Autodesk Inventor part; units mm, degrees
ref_plane "Work Plane1" through (-56.3599, 0, 22) normal (0, 0, -1) x (-1, 0, 0)
ref_plane "YZ Plane" through (0, 0, 0) normal (1, 0, 0) x (0, 1, 0)
ref_plane "XZ Plane" through (0, 0, 0) normal (0, 1, 0) x (-1, 0, 0)
ref_plane "Work Plane1" through (-56.3599, 0, 22) normal (0, 0, -1) x (-1, 0, 0)
sketch "Sketch1" plane through (-56.3599, 0, 22) normal (0, 0, -1) x (-1, 0, 0)
  line L0 (-4.0299, -0.3538) -> (-2.2322, 1.4439) construction
  arc A0 (-1.4439, 2.2322) -> (-2.2322, 1.4439) centre (-0.9299, 0.9299) ccw construction
  line L1 (-1.4439, 2.2322) -> (0.3538, 4.0299) construction
  line L2 (-37.8299, 42.8299) -> (-37.8299, 37.8299) construction
  line L3 (-37.8299, 37.8299) -> (-42.9208, 37.8299) construction
  line L4 (-37.8299, 42.2137) -> (-37.8299, 45.8299) construction
  line L5 (-37.8299, 45.8299) -> (-4.0299, 45.8299) construction
  line L6 (-4.0299, 45.8299) -> (-4.0299, 42.2137) construction
  line L7 (-4.0299, 4.0299) -> (0.3538, 4.0299)
  circle A1 centre (-20.9299, 20.9299) radius 17.5
  line L8 (-20.9299, 58.9723) -> (17.1124, 20.9299) construction
  line L9 (17.1124, 20.9299) -> (-20.9299, -17.1124) construction
  line L10 (-20.9299, -17.1124) -> (-58.9723, 20.9299) construction
  line L11 (-58.9723, 20.9299) -> (-20.9299, 58.9723) construction
  line L12 (-20.9299, 58.9723) -> (-20.9299, -17.1124) construction
  line L13 (17.1124, 20.9299) -> (-58.9723, 20.9299) construction
  line L14 (-20.9299, 58.9723) -> (32.8701, 58.9723) construction
  line L15 (-43.4299, 43.4299) -> (1.5701, 43.4299) construction
  line L16 (1.5701, 43.4299) -> (1.5701, -1.5701) construction
  line L17 (1.5701, -1.5701) -> (-43.4299, -1.5701) construction
  line L18 (-43.4299, -1.5701) -> (-43.4299, 43.4299) construction
  line L19 (-43.4299, 43.4299) -> (1.5701, -1.5701) construction
  line L20 (1.5701, 43.4299) -> (-43.4299, -1.5701) construction
  line L21 (-43.4299, 5.3876) -> (-43.4299, 36.4723)
  line L22 (-43.4299, 36.4723) -> (-36.4723, 43.4299)
  line L23 (-36.4723, 43.4299) -> (-5.3876, 43.4299)
  line L24 (-5.3876, 43.4299) -> (1.5701, 36.4723)
  line L25 (1.5701, 36.4723) -> (1.5701, 5.3876)
  line L26 (1.5701, 5.3876) -> (-5.3876, -1.5701)
  line L27 (-5.3876, -1.5701) -> (-36.4723, -1.5701)
  line L28 (-36.4723, -1.5701) -> (-43.4299, 5.3876)
  line L29 (-4.0299, 42.2137) -> (-37.8299, 42.2137)
  line L30 (-4.0299, -0.3538) -> (-4.0299, 4.0299)
  circle A2 centre (-20.9299, 20.9299) radius 1.5
  line L31 (-10.9299, 10.9299) -> (-30.9299, 10.9299) construction
  line L32 (-30.9299, 10.9299) -> (-30.9299, 30.9299) construction
  line L33 (-30.9299, 30.9299) -> (-10.9299, 30.9299) construction
  line L34 (-10.9299, 30.9299) -> (-10.9299, 10.9299) construction
  line L35 (-10.9299, 10.9299) -> (-30.9299, 30.9299) construction
  line L36 (-30.9299, 10.9299) -> (-10.9299, 30.9299) construction
  circle A3 centre (-30.9299, 30.9299) radius 1.4
  circle A4 centre (-30.9299, 10.9299) radius 1.4
  circle A5 centre (-10.9299, 10.9299) radius 1.4
  line L37 (-45.8299, 37.8299) -> (-42.0723, 37.8299) construction
  line L38 (-42.1723, 37.7299) -> (-45.8299, 37.7299)
  line L39 (-45.8299, 37.7299) -> (-45.8299, 4.1299)
  line L40 (-45.8299, 4.1299) -> (-42.1723, 4.1299)
  line L41 (-42.1723, 4.1299) -> (-42.1723, 37.7299)
  line L42 (-45.8299, 4.0299) -> (-42.0723, 4.0299) construction
  line L43 (-45.8299, 37.8299) -> (-42.0723, 37.8299)
  line L44 (-37.7299, 45.8299) -> (-4.1299, 45.8299)
  line L45 (-4.1299, 45.8299) -> (-4.1299, 42.1723)
  line L46 (-4.1299, 42.1723) -> (-37.7299, 42.1723)
  line L47 (-37.7299, 42.1723) -> (-37.7299, 45.8299)
  line L48 (0.4701, 37.8299) -> (0.4701, 4.0299) construction
  line L49 (0.4701, 4.0299) -> (3.9701, 4.0299) construction
  line L50 (3.9701, 37.8299) -> (3.9701, 4.0299) construction
  line L51 (0.4701, 37.8299) -> (3.9701, 37.8299) construction
  line L52 (-45.8299, -3.9701) -> (-4.0299, -3.9701) construction
  line L53 (0.3124, 37.7299) -> (3.9701, 37.7299)
  line L54 (3.9701, 37.7299) -> (3.9701, 4.1299)
  line L55 (3.9701, 4.1299) -> (0.3124, 4.1299)
  line L56 (0.3124, 4.1299) -> (0.3124, 37.7299)
  line L57 (-4.1713, -0.3538) -> (-37.7299, -0.3538)
  line L58 (-37.7299, -0.3538) -> (-37.7299, -3.9701)
  line L59 (-37.7299, -3.9701) -> (-4.1713, -3.9701)
  line L60 (-4.1713, -3.9701) -> (-4.1713, -0.3538)
  point P0 (-37.8299, 4.0299)
  dimension "d18" = 53.8
  dimension "d19" = 45
  dimension "d20" = 53.8
  dimension "d21" = 45
  dimension "d22" = 45
  dimension "d30" = 20
  dimension "d31" = 20
  dimension "d32" = 2.8
  dimension "d33" = 2.8
  dimension "d34" = 2.8
  dimension "d35" = 3
  dimension "d36" = 0.1
  dimension "d37" = 0.1
  dimension "d38" = 0.1
  dimension "d39" = 0.1
extrude "Extrusion1" add sketch "Sketch1" along normal blind 8 contours L30 L26 L57 L28 L41 L22 L46 L24 L56 L7 | L7 L26 L30 | L56 L24 L25 L26 | L26 L25 L24 L53 L54 L55 | L60 L59 L58 L57 L28 L27 L26 | L26 L27 L28 L57 | L46 L22 L29 L24 | L24 L29 L45 | L40 L39 L38 L22 L21 L28 | L28 L21 L22 L41 | L29 L22 L23 L24 | L24 L23 L22 L29 L47 L44 L45 | L47 L29 L22 | A1 | A2 | A3 | A4 | A5
sketch "Skizze4" plane through (-56.3599, 0, 14) normal (0, 0, -1) x (-1, 0, 0)
  line L0 (-37.7299, 42.1723) -> (-42.1723, 37.7299)
  line L1 (-42.1723, 37.7299) -> (-45.8299, 37.7299)
  line L2 (-45.8299, 37.7299) -> (-45.8299, 4.1299) construction
  line L3 (-45.8299, 4.1299) -> (-42.1723, 4.1299)
  line L4 (-42.1723, 4.1299) -> (-37.6885, -0.3538)
  line L5 (-37.6885, -0.3538) -> (-37.7299, -0.3538)
  line L6 (-37.7299, -0.3538) -> (-37.7299, -3.9701)
  line L7 (-37.7299, -3.9701) -> (-4.1713, -3.9701) construction
  line L8 (-4.1713, -3.9701) -> (-4.1713, -0.3538)
  line L9 (-4.1713, -0.3538) -> (0.3124, 4.1299)
  line L10 (0.3124, 4.1299) -> (3.9701, 4.1299)
  line L11 (3.9701, 4.1299) -> (3.9701, 37.7299) construction
  line L12 (3.9701, 37.7299) -> (0.3124, 37.7299)
  line L13 (0.3124, 37.7299) -> (-4.1299, 42.1723)
  line L14 (-4.1299, 42.1723) -> (-4.1299, 45.8299)
  line L15 (-4.1299, 45.8299) -> (-37.7299, 45.8299) construction
  line L16 (-37.7299, 45.8299) -> (-37.7299, 42.1723)
  line L17 (-37.9299, 46.0299) -> (-3.9299, 46.0299) construction
  line L18 (-3.9299, 46.0299) -> (-3.9299, 42.2551)
  line L19 (-3.9299, 42.2551) -> (0.3953, 37.9299)
  line L20 (0.3953, 37.9299) -> (4.1701, 37.9299)
  line L21 (4.1701, 37.9299) -> (4.1701, 3.9299) construction
  line L22 (4.1701, 3.9299) -> (0.3953, 3.9299)
  line L23 (0.3953, 3.9299) -> (-3.9713, -0.4367)
  line L24 (-3.9713, -0.4367) -> (-3.9713, -4.1701)
  line L25 (-3.9713, -4.1701) -> (-37.9299, -4.1701) construction
  line L26 (-37.9299, -4.1701) -> (-37.9299, -0.3953)
  line L27 (-37.9299, -0.3953) -> (-42.2551, 3.9299)
  line L28 (-42.2551, 3.9299) -> (-46.0299, 3.9299)
  line L29 (-46.0299, 3.9299) -> (-46.0299, 37.9299) construction
  line L30 (-46.0299, 37.9299) -> (-42.2551, 37.9299)
  line L31 (-42.2551, 37.9299) -> (-37.9299, 42.2551)
  line L32 (-37.9299, 42.2551) -> (-37.9299, 46.0299)
  line L33 (-45.8299, 37.7299) -> (-45.8299, 37.9299)
  line L34 (-4.1299, 45.8299) -> (-37.7299, 45.8299)
  line L35 (-37.7299, 45.8299) -> (-37.9299, 45.8299)
  line L36 (-4.1299, 45.8299) -> (-3.9299, 45.8299)
  line L37 (3.9701, 37.7299) -> (3.9701, 37.9299)
  line L38 (3.9701, 4.1299) -> (3.9701, 37.7299)
  line L39 (3.9701, 4.1299) -> (3.9701, 3.9299)
  line L40 (-4.1713, -3.9701) -> (-3.9713, -3.9701)
  line L41 (-37.7299, -3.9701) -> (-37.9299, -3.9701)
  line L42 (-45.8299, 4.1299) -> (-45.8299, 3.9299)
  point P0 (-56.3599, 0)
  dimension "d40" = 0.2
extrude "IM_offset" add sketch "Skizze4" against normal up to surface (8 mm away)
ref_plane "Arbeitsebene5" through (-35.4299, 3.9299, 22) normal (-1, 0, 0) x (0, 0, 1)
ref_plane "Arbeitsebene6" through (-18.4299, 20.9299, 22) normal (0, 1, 0) x (-1, 0, 0)
sketch "Sketch33" plane through (-56.3599, 0, 14) normal (0, 0, -1) x (-1, 0, 0)
  circle A0 centre (-20.9299, 20.9299) radius 15.24 construction
  circle A1 centre (-20.9299, 20.9299) radius 15.14 construction
  line L0 (-12.0272, 5.7899) -> (-29.8327, 5.7899)
  line L1 (-38.4929, 20.7899) -> (-29.5902, 36.2099)
  line L2 (-12.2697, 36.2099) -> (-3.3669, 20.7899)
  line L3 (-42.2551, 3.9299) -> (-45.8299, 3.9299)
  arc A2 (-12.0272, 5.7899) -> (-3.3669, 20.7899) centre (-12.0272, 15.7899) ccw
  arc A3 (-38.4929, 20.7899) -> (-29.8327, 5.7899) centre (-29.8327, 15.7899) ccw
  arc A4 (-12.2697, 36.2099) -> (-29.5902, 36.2099) centre (-20.9299, 31.2099) ccw
  point P0 (-56.3599, 0)
  point P1 (5.2933, 5.7899)
  point P2 (-47.1532, 5.7899)
  point P3 (-20.9299, 51.2099)
  dimension "d184" = 0.1
  dimension "d185" = 0
  dimension "d186" = 10
extrude "Extrusion27" cut sketch "Sketch33" against normal blind 10
sketch "Sketch34" plane through (-56.3599, 0, 22) normal (0, 0, 1) x (1, 0, 0)
  arc A0 (29.8327, 5.7899) -> (38.4929, 20.7899) centre (29.8327, 15.7899) ccw
  line L0 (29.8327, 5.7899) -> (12.0272, 5.7899)
  arc A1 (3.3669, 20.7899) -> (12.0272, 5.7899) centre (12.0272, 15.7899) ccw
  line L1 (3.3669, 20.7899) -> (12.2697, 36.2099)
  arc A2 (29.5902, 36.2099) -> (12.2697, 36.2099) centre (20.9299, 31.2099) ccw
  line L2 (29.5902, 36.2099) -> (38.4929, 20.7899)
  line L3 (3.9713, -3.9701) -> (37.9299, -3.9701)
  line L4 (37.9299, -3.9701) -> (37.9299, -0.3953)
  line L5 (37.9299, -0.3953) -> (42.2551, 3.9299)
  line L6 (42.2551, 3.9299) -> (45.8299, 3.9299)
  line L7 (45.8299, 3.9299) -> (45.8299, 37.9299)
  line L8 (45.8299, 37.9299) -> (42.2551, 37.9299)
  line L9 (42.2551, 37.9299) -> (37.9299, 42.2551)
  line L10 (37.9299, 42.2551) -> (37.9299, 45.8299)
  line L11 (37.9299, 45.8299) -> (3.9299, 45.8299)
  line L12 (3.9299, 45.8299) -> (3.9299, 42.2551)
  line L13 (3.9299, 42.2551) -> (-0.3953, 37.9299)
  line L14 (-0.3953, 37.9299) -> (-3.9701, 37.9299)
  line L15 (-3.9701, 37.9299) -> (-3.9701, 3.9299)
  line L16 (-3.9701, 3.9299) -> (-0.3953, 3.9299)
  line L17 (-0.3953, 3.9299) -> (3.9713, -0.4367)
  line L18 (3.9713, -0.4367) -> (3.9713, -3.9701)
  circle A3 centre (20.9299, 20.9299) radius 13.5001 construction
  circle A4 centre (20.9299, 20.9299) radius 13.4001
  line L19 (12.0272, 7.5298) -> (29.8327, 7.5298)
  arc A5 (29.8327, 7.5298) -> (36.9861, 19.92) centre (29.8327, 15.7899) ccw
  line L20 (36.9861, 19.92) -> (28.0834, 35.34)
  arc A6 (28.0834, 35.34) -> (13.7765, 35.34) centre (20.9299, 31.2099) ccw
  line L21 (13.7765, 35.34) -> (4.8737, 19.92)
  arc A7 (4.8737, 19.92) -> (12.0272, 7.5298) centre (12.0272, 15.7899) ccw
  point P0 (56.3599, 0)
  dimension "d189" = 0.1
extrude "Extrusion28" add sketch "Sketch34" along normal blind 1.5 contours L0 A1 L1 A2 L2 A0 | L18 L17 L16 L15 L14 L13 L12 L11 L10 L9 L8 L7 L6 L5 L4 L3
sketch "Sketch35" plane through (-52.3885, -3.9701, 14) normal (0, -1, 0) x (1, 0, 0)
  line L0 (0, 0) -> (0, 9.5)
  line L1 (0, 0) -> (33.9586, 0)
  line L2 (33.9586, 0) -> (33.9586, 9.5)
  line L3 (0, 9.5) -> (33.9586, 9.5)
  circle A0 centre (16.9586, 4.104) radius 1.4
  point P0 (52.3885, -14)
  dimension "d192" = 2.8
extrude "Extrusion29" cut sketch "Sketch35" along normal mid plane 30 contours A0
pattern_circular "Circular Pattern2" count 3 over 360 about axis through (-35.4299, 20.9299, 22) along (0, 0, 1) of "Extrusion29"
properties part number "20_Cube_Insert_Filter_25mm"
Input: part model. Units: mm. Frame: model coordinates. A direction names the side the tool comes from. Give positions to 0.01 mm unless a question says otherwise; leave off trailing zeros. Order: outer loops, then holes, each group sorted by start corner. A loop starts at its lowest first (then second) coordinate and runs counter-clockwise, first axis right, second up.
1. Draft query along Y for faces 6 (the face through (-23.76, 27.52, 22.74)), 7 (the face through (-59, 3.93, 19)), 8 (the face through (-51.425, 11.555, 22.74)), 9 (the face through (-59, 37.93, 19)). Return one class per face: released by +Y, released by -Y, zero draft, split by the parting line, or undercut.
Computed:
face 6: undercut
face 7: released by -Y
face 8: undercut
face 9: released by +Y
2. Cut plane B-B (x = -27.5). Return loops of the section in (y, z), and give its area (3 significant figures).
Computed:
outline: (-3.97, 14) - (5.79, 14) - (5.79, 22) - (7.53, 22) - (7.53, 23.5) - (-3.97, 23.5) - close; (34, 22) - (37.3, 22) - (37.3, 14) - (45.83, 14) - (45.83, 23.5) - (34, 23.5) - close
area: 181 mm2
3. Line query: probe 1 along Z at (x, y) = (-35.5, 4); probe 2 along Y at (x, z) = (-42.5, 17.75); probe 3 along Y at (x, z) = (-41, 22.5). Output: solid intervals per line, ascending.
Computed:
probe 1: z = 14 to 16.71, 19.5 to 23.5
probe 2: y = -3.97 to 5.79, 38.28 to 45.83
probe 3: y = -3.97 to 7.53, 37.31 to 45.83
4. Pin query (flat end, axial travel): pin 1 Ø4 at (y, z) = (43.5, 20) entering from -X; pin 2 Ø1.8 at (x, z) = (-58, 18) entering from -Y; pin 3 Ø1.8 at (y, z) = (-1.5, 20.5) entering from +X. Return the tip coordinate at first contact, or that it passes through.
Computed:
pin 1: stops at x = -53.19
pin 2: stops at y = 3.93
pin 3: stops at x = -18.43
5. Cut plane D-D (x = -20). State how many separate pieces and enclosed holes the cut face has, and give its area (3 significant figures).
Computed:
separate pieces: 2
enclosed holes: 1
area: 320 mm2
6. Cut plane C-C (y = 8.5). Return loops of the section in (x, z), and give its area (3 significant figures).
Computed:
outline: (-60.33, 14) - (-51.18, 14) - (-51.18, 22) - (-48.22, 22) - (-48.22, 23.5) - (-60.33, 23.5) - close; (-22.64, 22) - (-19.68, 22) - (-19.68, 14) - (-10.53, 14) - (-10.53, 23.5) - (-22.64, 23.5) - close
area: 183 mm2
7. Set-up query: faces 1 (the face through (-22.256, 28.392, 19.722)), 2 (the face through (-35, -3.97, 20)), 3 (the face through (-12, 37.93, 19)), 4 (the face through (-52.389, -2, 19)), 5 (the face through (-19.31, 11.77, 22.74)). Return all of +Z, -Z, +X, -X, +Y, -Y with unobstructed straight access to the full face (end or side cutting, diameter ignored); none if empty.
Computed:
face 1: -Z
face 2: +Z, -Z, +X, -X, -Y
face 3: +Z, -Z, +X, +Y
face 4: +Z, -Z, -X, -Y
face 5: +Z, -Z
8. Cut plane A-A (z = 21.25). Return loops of the section in (x, y), and give its area (3 significant figures).
Computed:
outline: (-60.33, 3.93) - (-56.76, 3.93) - (-52.39, -0.44) - (-52.39, -3.97) - (-18.43, -3.97) - (-18.43, -0.4) - (-14.1, 3.93) - (-10.53, 3.93) - (-10.53, 37.93) - (-14.1, 37.93) - (-18.43, 42.26) - (-18.43, 45.83) - (-52.43, 45.83) - (-52.43, 42.26) - (-56.76, 37.93) - (-60.33, 37.93) - close; hole (-52.99, 20.79) arc R10 ccw to (-44.33, 5.79) - (-26.53, 5.79) arc R10 ccw to (-17.87, 20.79) - (-26.77, 36.21) arc R10 ccw to (-44.09, 36.21) - close
area: 1,280 mm2
